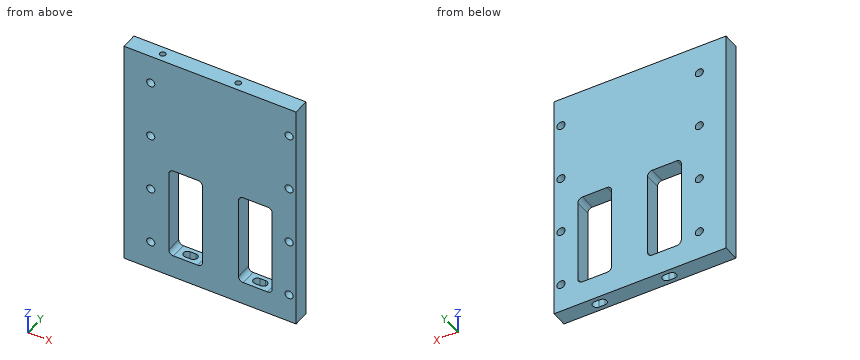
```python
from build123d import *

# Parameters (mm, degrees)
BOSS_EXTRUDE1_DEPTH       = 200
CUT_EXTRUDE1_DEPTH        = 250.198715888
F_6_0MM_DOWEL_SLOT1_DEPTH = 20
M6X1_0_TAPPED_HOLE1_D     = 5
M6X1_0_TAPPED_HOLE1_DEPTH = 21.497848452
M6X1_0_TAPPED_HOLE1_TIP   = 1.502151548
FILLET1_R                 = 4
BOSS_EXTRUDE2_DEPTH       = 80
FILLET2_R                 = 4
SKETCH13_R                = 3.5
CUT_EXTRUDE2_DEPTH        = 250.198715888


# Read off the part's stored shape, not the designer's step: Ø6.0mm Dowel Slot1
with BuildPart() as part:
    # Sketch1 → Boss-Extrude1 (new body)
    with BuildSketch(Plane.XY):
        Polygon((-21, 207), (-148, 207), (-148, 197.5), (-148, 193), (-24, 193), (-12, 193), (0, 193), (0, 207), (-12, 207), align=None)
    extrude(amount=BOSS_EXTRUDE1_DEPTH)

    # Sketch3 → Cut-Extrude1 (cut, through all)
    with BuildSketch(Plane(origin=(0, 207, 0), x_dir=(1, 0, 0), z_dir=(0, 1, 0))):
        Polygon((-20.5, -100), (-20.5, -20), (-22.5, -20), (-27.5, -20), (-39.5, -20), (-42, -20), (-107.5, -20), (-109.5, -20), (-109.5, -100), (-107.5, -100), (-42, -100), (-39.5, -100), (-27.5, -100), (-22.5, -100), align=None)
    extrude(amount=-CUT_EXTRUDE1_DEPTH, mode=Mode.SUBTRACT)

    # Ø6.0mm Dowel Slot1 outline → Ø6.0mm Dowel Slot1 (cut)
    with BuildSketch(Plane.XY):
        with BuildLine():
            Line((-37.5, 196.5), (-32.5, 196.5))
            ThreePointArc((-32.5, 196.5), (-29, 200), (-32.5, 203.5))
            Line((-32.5, 203.5), (-37.5, 203.5))
            ThreePointArc((-37.5, 203.5), (-41, 200), (-37.5, 196.5))
        make_face()
        with BuildLine():
            ThreePointArc((-92.5, 196.5), (-89, 200), (-92.5, 203.5))
            Line((-92.5, 203.5), (-97.5, 203.5))
            ThreePointArc((-97.5, 203.5), (-101, 200), (-97.5, 196.5))
            Line((-97.5, 196.5), (-92.5, 196.5))
        make_face()
    extrude(amount=F_6_0MM_DOWEL_SLOT1_DEPTH, mode=Mode.SUBTRACT)

    # M6x1.0 Tapped Hole1
    with Locations(Plane.XY.offset(200)):
        with Locations((-119, 200), (-54, 200)):
            Hole(M6X1_0_TAPPED_HOLE1_D / 2, depth=M6X1_0_TAPPED_HOLE1_DEPTH)
            with Locations((0, 0, -(M6X1_0_TAPPED_HOLE1_DEPTH + M6X1_0_TAPPED_HOLE1_TIP / 2))):  # 118° drill point
                Cone(0, M6X1_0_TAPPED_HOLE1_D / 2, M6X1_0_TAPPED_HOLE1_TIP, mode=Mode.SUBTRACT)

    # Fillet1
    fillet1_edges = [part.edges().sort_by_distance(p)[0] for p in [
        (-20.5, 200, 100),
        (-109.5, 200, 100),
        (-109.5, 200, 20),
        (-20.5, 200, 20),
    ]]
    fillet(fillet1_edges, radius=FILLET1_R)

    # Sketch15 → Boss-Extrude2 (add)
    with BuildSketch(Plane.XY.offset(20)):
        Polygon((-80.5, 200), (-80.5, 193), (-49.5, 193), (-49.5, 200), (-49.5, 207), (-80.5, 207), align=None)
    extrude(amount=BOSS_EXTRUDE2_DEPTH)

    # Fillet2
    fillet2_edges = [part.edges().sort_by_distance(p)[0] for p in [
        (-80.5, 200, 20),
        (-49.5, 200, 20),
        (-80.5, 200, 100),
        (-49.5, 200, 100),
    ]]
    fillet(fillet2_edges, radius=FILLET2_R)

    # Sketch13 → Cut-Extrude2 (cut, through all)
    with BuildSketch(Plane.XZ.offset(-193)):
        with Locations(Location((-6, 75, 0), (0, 0, 270))):
            Circle(SKETCH13_R)
        with Locations(Location((-6, 125, 0), (0, 0, 270))):
            Circle(SKETCH13_R)
        with Locations(Location((-6, 175, 0), (0, 0, 270))):
            Circle(SKETCH13_R)
        with Locations(Location((-125, 125, 0), (0, 0, 270))):
            Circle(SKETCH13_R)
        with Locations(Location((-125, 75, 0), (0, 0, 270))):
            Circle(SKETCH13_R)
        with Locations(Location((-6, 25, 0), (0, 0, 270))):
            Circle(SKETCH13_R)
        with Locations(Location((-125, 175, 0), (0, 0, 270))):
            Circle(SKETCH13_R)
        with Locations(Location((-125, 25, 0), (0, 0, 270))):
            Circle(SKETCH13_R)
    extrude(amount=-CUT_EXTRUDE2_DEPTH, mode=Mode.SUBTRACT)


solid = part.part
```
Part model, mm, in its own coordinate system. Round coordinates to 2 decimals unless told otherwise and drop trailing zeros. Write each loop counter-clockwise with the first axis right and the second up, starting at its lowest first coordinate (ties: lowest second). Pieces come first, ordered by that corner, then holes.
Item 1: Cut at C-C, the plane z = 75. Give the cut face in (x, y).
Results:
outline: (-148, 193) - (-128.5, 193) - (-128.5, 207) - (-148, 207) - close; (-121.5, 193) - (-109.5, 193) - (-109.5, 207) - (-121.5, 207) - close; (-80.5, 193) - (-49.5, 193) - (-49.5, 207) - (-80.5, 207) - close; (-20.5, 193) - (-9.5, 193) - (-9.5, 207) - (-20.5, 207) - close; (-2.5, 193) - (0, 193) - (0, 207) - (-2.5, 207) - close
Item 2: Drop a flat-ended pin along its axis: pin 1 Ø5.5 at (x, z) = (-125, 175) entering from -Y. Give the stop position or say it passes through.
Results:
pin 1: passes through
Item 3: Cut at B-B, the plane x = -6. Give the cut face in (y, z), plus the area to 3 significant figures.
Results:
outline: (193, 0) - (207, 0) - (207, 21.5) - (193, 21.5) - close; (193, 28.5) - (207, 28.5) - (207, 71.5) - (193, 71.5) - close; (193, 78.5) - (207, 78.5) - (207, 121.5) - (193, 121.5) - close; (193, 128.5) - (207, 128.5) - (207, 171.5) - (193, 171.5) - close; (193, 178.5) - (207, 178.5) - (207, 200) - (193, 200) - close
area: 2,410 mm2
Item 4: Cut at A-A, the plane z = 49. Give the cut face in (x, y).
Results:
outline: (-148, 193) - (-109.5, 193) - (-109.5, 207) - (-148, 207) - close; (-80.5, 193) - (-49.5, 193) - (-49.5, 207) - (-80.5, 207) - close; (-20.5, 193) - (0, 193) - (0, 207) - (-20.5, 207) - close
Item 5: Probe L1, parallel to X at y = 202.75, z = 35.5; L2, parallel to X at y = 199.25, z = 175; L3, parallel to Y at x = -54, z = 189. List the from-to ranges inside material, lowest first.
Results:
L1: x = -148 to -109.5, -80.5 to -49.5, -20.5 to 0
L2: x = -148 to -128.5, -121.5 to -9.5, -2.5 to 0
L3: y = 193 to 197.5, 202.5 to 207
Item 6: Cut at D-D, the plane z = 125. Give the cut face in (x, y), plus the area to 3 significant figures.
Results:
outline: (-148, 193) - (-128.5, 193) - (-128.5, 207) - (-148, 207) - close; (-121.5, 193) - (-9.5, 193) - (-9.5, 207) - (-121.5, 207) - close; (-2.5, 193) - (0, 193) - (0, 207) - (-2.5, 207) - close
area: 1,880 mm2
